from build123d import *

# Parameters (mm, degrees)
CROQUIS1_R              = 1.5
SALIENTE_EXTRUIR1_DEPTH = 10
CROQUIS2_W              = 8
CROQUIS2_H              = 7.5
CROQUIS2_W_2            = 15
CROQUIS2_H_2            = 8
CROQUIS2_W_3            = 9
CORTAR_EXTRUIR1_DEPTH   = 2.75
REDONDEO1_R             = 1


with BuildPart() as part:
    # Croquis1 → Saliente-Extruir1 (new, symmetric)
    with BuildSketch(Plane(origin=(0, 0, 0), x_dir=(0, 0, -1), z_dir=(1, 0, 0))):
        with BuildLine():
            Line((-15, 4), (-1, 4))
            Line((-1, 4), (-1, 16))
            ThreePointArc((-1, 16), (3, 20), (7, 16))
            Line((7, 16), (7, 4))
            Line((7, 4), (15, 4))
            ThreePointArc((15, 4), (19, 0), (15, -4))
            Line((15, -4), (-15, -4))
            Line((-15, -4), (-38, -4))
            ThreePointArc((-38, -4), (-42, 0), (-38, 4))
            Line((-38, 4), (-15, 4))
        make_face()
        with Locations((15, 0)):
            Circle(CROQUIS1_R, mode=Mode.SUBTRACT)
        with Locations((3, 16)):
            Circle(CROQUIS1_R, mode=Mode.SUBTRACT)
        with Locations((-15, 0)):
            Circle(CROQUIS1_R, mode=Mode.SUBTRACT)
        with Locations((-38, 0)):
            Circle(CROQUIS1_R, mode=Mode.SUBTRACT)
    extrude(amount=SALIENTE_EXTRUIR1_DEPTH, both=True)

    # Croquis2 → Cortar-Extruir1 (cut, symmetric)
    with BuildSketch(Plane(origin=(0, 0, 0), x_dir=(0, 0, -1), z_dir=(1, 0, 0))):
        with Locations((3, 16.25)):
            Rectangle(CROQUIS2_W, CROQUIS2_H)
        with Locations((-15.5, 0)):
            Rectangle(CROQUIS2_W_2, CROQUIS2_H_2)
        with Locations((14.5, 0)):
            Rectangle(CROQUIS2_W_3, CROQUIS2_H_2)
        with Locations((-37.5, 0)):
            Rectangle(CROQUIS2_W_3, CROQUIS2_H_2)
    extrude(amount=CORTAR_EXTRUIR1_DEPTH, both=True, mode=Mode.SUBTRACT)

    # Redondeo1
    redondeo1_edges = [part.edges().sort_by_distance(p)[0] for p in [
        (2.75, 0, -10),
        (-2.75, 0, -10),
        (-2.75, 0, 23),
        (2.75, 0, 23),
        (2.75, 0, 33),
        (-2.75, 0, 33),
    ]]
    fillet(redondeo1_edges, radius=REDONDEO1_R)


solid = part.part
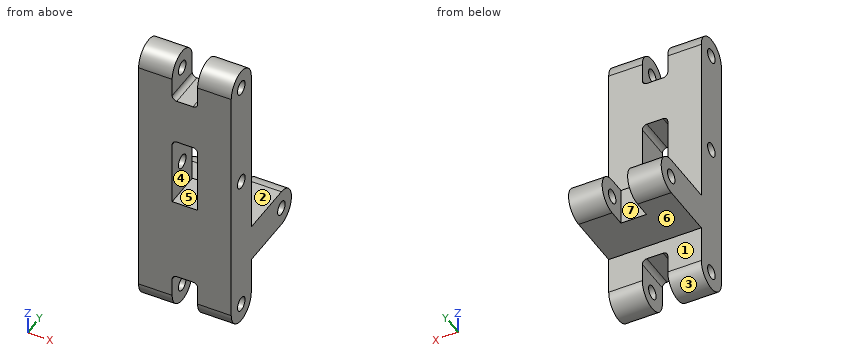
The listing builds one solid part. Answer for the finished solid, in the listing's coordinates (mm). Face numbers are marked on the shaded views. A direction names the side the tool comes from. Give positions to 0.01 mm unless a question says otherwise; leave off trailing zeros. Loops run counter-clockwise (first coordinate to the right, second up) from the corner with the lowest first, then second, coordinate; pieces in that order, holes last.
Item 1: A cutting plane is placed at D-D (x = -1). Give the vertices of the cut face in (y, z), then the cut area to 3 significant figures.
Derived:
outline: (-4, -10) - (4, -10) - (4, -7) - (12.5, -7) - (12.5, 1) - (4, 1) - (4, 8) - (-4, 8) - close; (-4, 23) - (4, 23) - (4, 33) - (-4, 33) - close
area: 292 mm2
Item 2: A cutting plane is placed at B-B (x = -8.5). Give the vertices of the cut face in (y, z).
Derived:
outline: (-4, -15) arc R4 ccw to (4, -15) - (4, -7) - (16, -7) arc R4 ccw to (16, 1) - (4, 1) - (4, 38) arc R4 ccw to (-4, 38) - close; hole circle Ø3 at (0, -15); hole circle Ø3 at (0, 15); hole circle Ø3 at (0, 38); hole circle Ø3 at (16, -3)
Item 3: A cutting plane is placed at A-A (z = 19.5). Give the vertices of the cut face in (x, y), then the cut area to 3 significant figures.
Derived:
outline: (-10, -4) - (-2.75, -4) - (-2.75, 4) - (-10, 4) - close; (2.75, -4) - (10, -4) - (10, 4) - (2.75, 4) - close
area: 116 mm2
Item 4: Each of these flat-tipped pins is pushed along its axis until it touches: pin 1 Ø4 at (y, z) = (0.5, 37.5) entering from +X; pin 2 Ø6 at (x, y) = (4, 9) entering from -Z; pin 3 Ø2 at (y, z) = (5.5, 19) entering from +X; pin 4 Ø9 at (x, z) = (4.5, -10) entering from +Y. Where does it stop, or does it pass through?
Derived:
pin 1: stops at x = 10
pin 2: stops at z = -7
pin 3: passes through
pin 4: stops at y = 19.12
Item 5: A cutting plane is placed at C-C (z = -3). Give the vertices of the cut face in (x, y).
Derived:
outline: (-10, -4) - (10, -4) - (10, 14.5) - (2.75, 14.5) - (2.75, 12.5) - (-2.75, 12.5) - (-2.75, 14.5) - (-10, 14.5) - close; (-10, 17.5) - (-2.75, 17.5) - (-2.75, 20) - (-10, 20) - close; (2.75, 17.5) - (10, 17.5) - (10, 20) - (2.75, 20) - close
Item 6: Determine the mould class of the marked faces 1, 2, 3 and 4 for opening direction Z: +Z half, -Z half, draft (parallel to the pull), parting line (faces both ways), or undercut.
Derived:
face 1: draft
face 2: +Z half
face 3: -Z half
face 4: undercut
Item 7: Find the intervals of material crossed by line 1 along Z through (x, y) = (4.5, 0); line 2 along X through (y, z) = (17.75, -0.5); line 3 along Y through (x, z) = (8, -3), in increasing order.
Derived:
line 1: z = -19 to -16.5, -13.5 to 13.5, 16.5 to 36.5, 39.5 to 42
line 2: x = -10 to -2.75, 2.75 to 10
line 3: y = -4 to 14.5, 17.5 to 20
Item 8: A tool of negligible diameter and unlimited length cuts with its end or side. For the marked faces 5, 6 and 7, from which of +Z, -Z, +X, -X, +Y, -Y can it reach the whole face along a straight path? Write none if from no direction.
Derived:
face 5: +Y, -Y
face 6: -Z, +X, -X, +Y
face 7: +Z, -Z, +Y
